from build123d import *

# Parameters (mm, degrees)
EXTRUDE_1_DEPTH       = 330
EXTRUDE_3_DEPTH       = 330
PATTERN_CURVE_1_DEPTH = 330
SKETCH_3_R            = 1.6
CUT_EXTRUDE_1_DEPTH   = 6


# Read off the part's stored shape, not the designer's step: the pattern curve step
with BuildPart() as part:
    # Sketch 1 → Extrude 1 (new body)
    with BuildSketch(Plane.XY):
        with BuildLine():
            Line((0, 40), (1.528979332, 40))
            ThreePointArc((1.528979332, 40), (2.225614441, 39.717425624), (2.528547087, 39.029399052))
            Line((2.528547087, 39.029399052), (3.5, 6))
            Line((3.5, 6), (118.5, 6))
            Line((118.5, 6), (119.471452913, 39.029399052))
            ThreePointArc((119.471452913, 39.029399052), (119.774385559, 39.717425624), (120.471020668, 40))
            Line((120.471020668, 40), (122, 40))
            Line((122, 40), (122, 0))
            Line((122, 0), (0, 0))
            Line((0, 0), (0, 40))
        make_face()
    extrude(amount=EXTRUDE_1_DEPTH)

    # Sketch 2 → Extrude 3 (add)
    with BuildSketch(Plane.XY.offset(330)):
        with BuildLine():
            Line((10.5, 39.5), (9.25, 6))
            Line((9.25, 6), (12.75, 6))
            Line((12.75, 6), (11.5, 39.5))
            ThreePointArc((11.5, 39.5), (11, 40), (10.5, 39.5))
        make_face()
    extrude(amount=-EXTRUDE_3_DEPTH)

    # Pattern Curve 1 outline → Pattern Curve 1 (add)
    with BuildSketch(Plane.XY):
        with BuildLine():
            ThreePointArc((21.5, 39.5), (21, 40), (20.5, 39.5))
            Line((20.5, 39.5), (19.25, 6))
            Line((19.25, 6), (22.75, 6))
            Line((22.75, 6), (21.5, 39.5))
        make_face()
        with BuildLine():
            Line((110.5, 39.5), (109.25, 6))
            Line((109.25, 6), (112.75, 6))
            Line((112.75, 6), (111.5, 39.5))
            ThreePointArc((111.5, 39.5), (111, 40), (110.5, 39.5))
        make_face()
        with BuildLine():
            Line((100.5, 39.5), (99.25, 6))
            Line((99.25, 6), (102.75, 6))
            Line((102.75, 6), (101.5, 39.5))
            ThreePointArc((101.5, 39.5), (101, 40), (100.5, 39.5))
        make_face()
        with BuildLine():
            Line((90.5, 39.5), (89.25, 6))
            Line((89.25, 6), (92.75, 6))
            Line((92.75, 6), (91.5, 39.5))
            ThreePointArc((91.5, 39.5), (91, 40), (90.5, 39.5))
        make_face()
        with BuildLine():
            Line((80.5, 39.5), (79.25, 6))
            Line((79.25, 6), (82.75, 6))
            Line((82.75, 6), (81.5, 39.5))
            ThreePointArc((81.5, 39.5), (81, 40), (80.5, 39.5))
        make_face()
        with BuildLine():
            Line((70.5, 39.5), (69.25, 6))
            Line((69.25, 6), (72.75, 6))
            Line((72.75, 6), (71.5, 39.5))
            ThreePointArc((71.5, 39.5), (71, 40), (70.5, 39.5))
        make_face()
        with BuildLine():
            Line((60.5, 39.5), (59.25, 6))
            Line((59.25, 6), (62.75, 6))
            Line((62.75, 6), (61.5, 39.5))
            ThreePointArc((61.5, 39.5), (61, 40), (60.5, 39.5))
        make_face()
        with BuildLine():
            Line((50.5, 39.5), (49.25, 6))
            Line((49.25, 6), (52.75, 6))
            Line((52.75, 6), (51.5, 39.5))
            ThreePointArc((51.5, 39.5), (51, 40), (50.5, 39.5))
        make_face()
        with BuildLine():
            Line((40.5, 39.5), (39.25, 6))
            Line((39.25, 6), (42.75, 6))
            Line((42.75, 6), (41.5, 39.5))
            ThreePointArc((41.5, 39.5), (41, 40), (40.5, 39.5))
        make_face()
        with BuildLine():
            Line((30.5, 39.5), (29.25, 6))
            Line((29.25, 6), (32.75, 6))
            Line((32.75, 6), (31.5, 39.5))
            ThreePointArc((31.5, 39.5), (31, 40), (30.5, 39.5))
        make_face()
    extrude(amount=PATTERN_CURVE_1_DEPTH)

    # Sketch 3 → Cut-Extrude 1 (cut)
    with BuildSketch(Plane.XZ):
        with Locations((28, 321.5)):
            Circle(SKETCH_3_R)
        with Locations((94, 321.5)):
            Circle(SKETCH_3_R)
        with Locations(Location((94, 8.5, 0), (0, 0, 218.624832873))):
            Circle(SKETCH_3_R)
        with Locations(Location((28, 8.5, 0), (0, 0, 38.624832873))):
            Circle(SKETCH_3_R)
    extrude(amount=-CUT_EXTRUDE_1_DEPTH, mode=Mode.SUBTRACT)


solid = part.part
The listing builds one solid part. Answer for the finished solid, in the listing's coordinates (mm). Coordinates: 2 decimals unless noted, no trailing zeros. Write each question's results on one line, items separated by ' | '.
Item 1: For a pull along X with two mould halves and no side action, classify faces 1 (the face through (26, 6, 163)), 2 (the face through (61, 13, 0)) as released by +X, released by -X, zero draft, split by the parting line, or undercut.
Answer below:
face 1: undercut | face 2: zero draft
Item 2: The part is cut by section A-A on y = 17. State how many separate pieces and enclosed holes the cut face has, and give its area (3 significant figures).
Answer below:
separate pieces: 13 | enclosed holes: 0 | area: 11,800 mm2
Item 3: Consider probe 1 along Z at (x, y) = (28, 1.3); probe 2 along X at (y, z) = (1.8, 8.5); probe 3 along X at (y, z) = (4, 8). Determine where each line is inside the solid, lowest interval first. Write a range as [from, to].
Answer below:
probe 1: [0, 6.9], [10.1, 319.9], [323.1, 330] | probe 2: [0, 26.4], [29.6, 92.4], [95.6, 122] | probe 3: [0, 26.48], [29.52, 92.48], [95.52, 122]
Item 4: Given P1, Ø1.9, axis at x = 28, z = 321.5, coming from the -Y side; P2, Ø2, axis at x = 106.5, z = 239, coming from the +Y side; P3, Ø1, axis at x = 76.5, z = 68, coming from the -Y side; P4, Ø6.5, axis at x = 5, z = 137.5, coming from the +Y side, each flat-ended and moving along its own axis, determine where each tip first touches the part or whether it passes through.
Answer below:
P1: through | P2: y = 6 | P3: y = 0 | P4: y = 39.98
